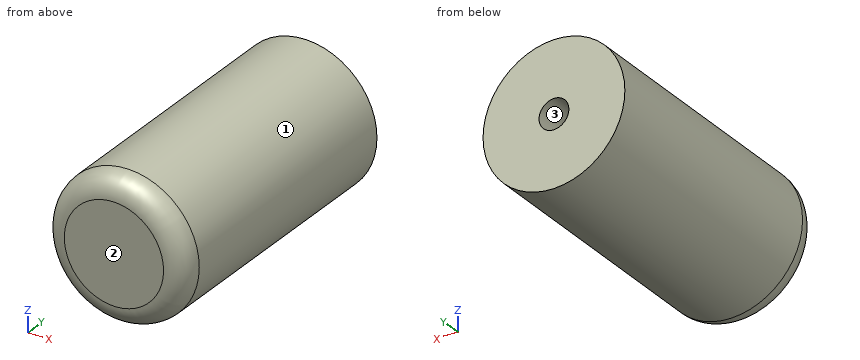
```python
from build123d import *

# Parameters (mm, degrees)
SKETCH1_R           = 10
BOSS_EXTRUDE1_DEPTH = 40
FILLET1_R           = 3
SKETCH3_R           = 2.1
CUT_EXTRUDE1_DEPTH  = 10


with BuildPart() as part:
    # Sketch1 → Boss-Extrude1 (new body)
    with BuildSketch(Plane(origin=(0, 0, 0), x_dir=(1, 0, 0), z_dir=(0, 1, 0))):
        Circle(SKETCH1_R)
    extrude(amount=BOSS_EXTRUDE1_DEPTH)

    # Fillet1
    fillet1_edges = [part.edges().sort_by_distance(p)[0] for p in [
        (-10, 0, 0),
    ]]
    fillet(fillet1_edges, radius=FILLET1_R)

    # Sketch3 → Cut-Extrude1 (cut)
    with BuildSketch(Plane(origin=(0, 40, 0), x_dir=(1, 0, 0), z_dir=(0, 1, 0))):
        Circle(SKETCH3_R)
    extrude(amount=-CUT_EXTRUDE1_DEPTH, mode=Mode.SUBTRACT)


solid = part.part
```
Part model, mm, in its own coordinate system. Face numbers are marked on the shaded views. Round coordinates to 2 decimals unless told otherwise and drop trailing zeros. Loops run counter-clockwise (first coordinate to the right, second up) from the corner with the lowest first, then second, coordinate; pieces in that order, holes last. Notation, with made-up numbers: (20, 46) -> (54, 46) arc R18 ccw to (54, 79) -> close; hole circle Ø5 at (68, 21). An arc over 180 degrees is marked (long way). Use a Markdown table: item, result.
1) Cut at C-C, the plane y = 21. List the corners of the cut face in (x, z), and give its area (3 significant figures).
The answers:
| item | result |
|---|---|
| outline | circle Ø20 at (0, 0) |
| area | 314 mm2 |
2) Cut at B-B, the plane y = 37. List the corners of the cut face in (x, z), and give its area (3 significant figures).
The answers:
| item | result |
|---|---|
| outline | circle Ø20 at (0, 0); hole circle Ø4.2 at (0, 0) |
| area | 300 mm2 |
3) Pull direction Z, two halves, no side cores. Call the marked faces 1, 2 and 3: pulls with the +Z half, pulls with the -Z half, needs draft (parallel to the pull), parting line crosses it, or undercut.
The answers:
| item | result |
|---|---|
| face 1 | parting line crosses it |
| face 2 | needs draft |
| face 3 | undercut |
4) Probe line 1 (Z direction, x = 0, y = 34.25); line 2 (Y direction, x = -0.25, z = -0.25). List the from-to ranges inside material, lowest first. Write a range as [from, to].
The answers:
| item | result |
|---|---|
| line 1 | z = [-10, -2.1], [2.1, 10] |
| line 2 | y = [0, 30] |
5) Cut at A-A, the plane z = 0. List the corners of the cut face in (x, y).
The answers:
| item | result |
|---|---|
| outline | (-10, 3) arc R3 ccw to (-7, 0) -> (7, 0) arc R3 ccw to (10, 3) -> (10, 40) -> (2.1, 40) -> (2.1, 30) -> (-2.1, 30) -> (-2.1, 40) -> (-10, 40) -> close |
6) Drop flat-ended pins along their axis: pin 1 Ø2.5 at (x, z) = (0, 0) entering from +Y; pin 2 Ø4 at (y, z) = (34, 6.5) entering from +X; pin 3 Ø6 at (y, z) = (22, -5.5) entering from -X. Give the stop position or say it passes through.
The answers:
| item | result |
|---|---|
| pin 1 | stops at y = 30 |
| pin 2 | stops at x = 8.93 |
| pin 3 | stops at x = -9.68 |
